Verification items for the finished model (mm, model axes). Face numbers are marked on the shaded views. A direction names the side the tool comes from. Give positions to 0.01 mm unless a question says otherwise; leave off trailing zeros. Loops run counter-clockwise (first coordinate to the right, second up) from the corner with the lowest first, then second, coordinate; pieces in that order, holes last. Notation, with made-up numbers: M 25,86.5 L 75,86.5 A17 ccw 75,113.5 Z; hole C 23,6.25 d11. An arc over 180 degrees is marked long. Answer in a Markdown table with one row per item.
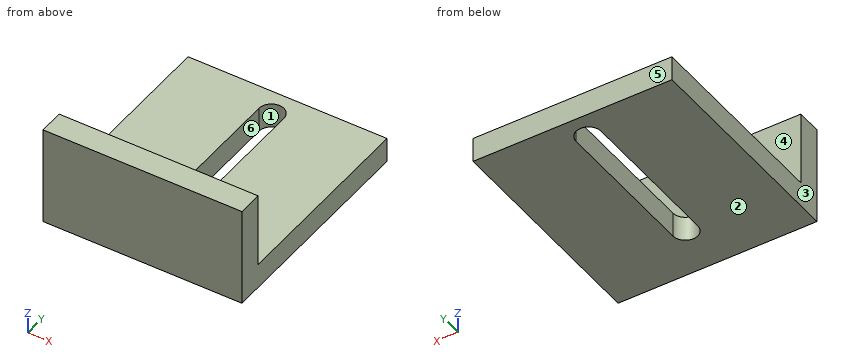
```python
from build123d import *

# Parameters (mm, degrees)
SKETCH1_W           = 25.4
SKETCH1_H           = 12.7
BOSS_EXTRUDE1_DEPTH = 3.175
SKETCH2_W           = 25.4
SKETCH2_H           = 3.175
BOSS_EXTRUDE2_DEPTH = 25.4
CUT_EXTRUDE1_DEPTH  = 33.688625698


with BuildPart() as part:
    # Sketch1 → Boss-Extrude1 (new body)
    with BuildSketch(Plane(origin=(0, 0, 0), x_dir=(1, 0, 0), z_dir=(0, 1, 0))):
        Rectangle(SKETCH1_W, SKETCH1_H)
    extrude(amount=BOSS_EXTRUDE1_DEPTH)

    # Sketch2 → Boss-Extrude2 (add)
    with BuildSketch(Plane(origin=(0, 3.175, 0), x_dir=(1, 0, 0), z_dir=(0, 1, 0))):
        with Locations((0, 4.7625)):
            Rectangle(SKETCH2_W, SKETCH2_H)
    extrude(amount=BOSS_EXTRUDE2_DEPTH)

    # Sketch3 → Cut-Extrude1 (cut, through all)
    with BuildSketch(Plane.XY.offset(-3.175)):
        with BuildLine():
            Line((1.5875, 25.4), (1.5875, 6.35))
            ThreePointArc((1.5875, 6.35), (0, 4.7625), (-1.5875, 6.35))
            Line((-1.5875, 6.35), (-1.5875, 25.4))
            ThreePointArc((-1.5875, 25.4), (0, 26.9875), (1.5875, 25.4))
        make_face()
    extrude(amount=-CUT_EXTRUDE1_DEPTH, mode=Mode.SUBTRACT)


solid = part.part
```
Item 1: Release check for a two-part mould opening along X. For the marked faces 1, 2 and 3 record: released by +X, released by -X, zero draft, split by the parting line, or undercut.
Reported:
| item | result |
|---|---|
| face 1 | undercut |
| face 2 | zero draft |
| face 3 | released by -X |
Item 2: Tool access check on the marked faces 4, 5 and 6. Record the directions out of +Z, -Z, +X, -X, +Y, -Y that give a thin tool (end or side, any length) a straight path to the whole face; none if there is none.
Reported:
| item | result |
|---|---|
| face 4 | +Z, +X, -X, +Y |
| face 5 | +Z, -Z, +X, -X, +Y |
| face 6 | +Z, -Z |
Item 3: Go/stop test with flat-tipped pins: pin 1 (6 mm diameter, centred on x = -2, y = 24, fed in from +Z) (3 decimals); pin 2 (7.5 mm diameter, centred on x = 4.5, z = 2.5, fed in from +Y) (3 decimals). Record where each tip stops, or that it passes through.
Reported:
| item | result |
|---|---|
| pin 1 | stops at z = -3.175 |
| pin 2 | stops at y = 3.175 |
Item 4: Sectioned sample at D-D (x = -6.75). Record the cut outline in (y, z) (3 decimals).
Reported:
| item | result |
|---|---|
| outline | M 0,-6.35 L 28.575,-6.35 L 28.575,-3.175 L 3.175,-3.175 L 3.175,6.35 L 0,6.35 Z |
Item 5: Scan lines: L1, parallel to X at y = 20.5, z = -4.75; L2, parallel to Y at x = -1.75, z = 2 (3 decimals); L3, parallel to Z at x = 9.25, y = 7.5 (3 decimals). Record each from-to range of solid material in increasing order. Write a range as [from, to].
Reported:
| item | result |
|---|---|
| L1 | x = [-12.7, -1.59], [1.59, 12.7] |
| L2 | y = [0, 3.175] |
| L3 | z = [-6.35, -3.175] |
